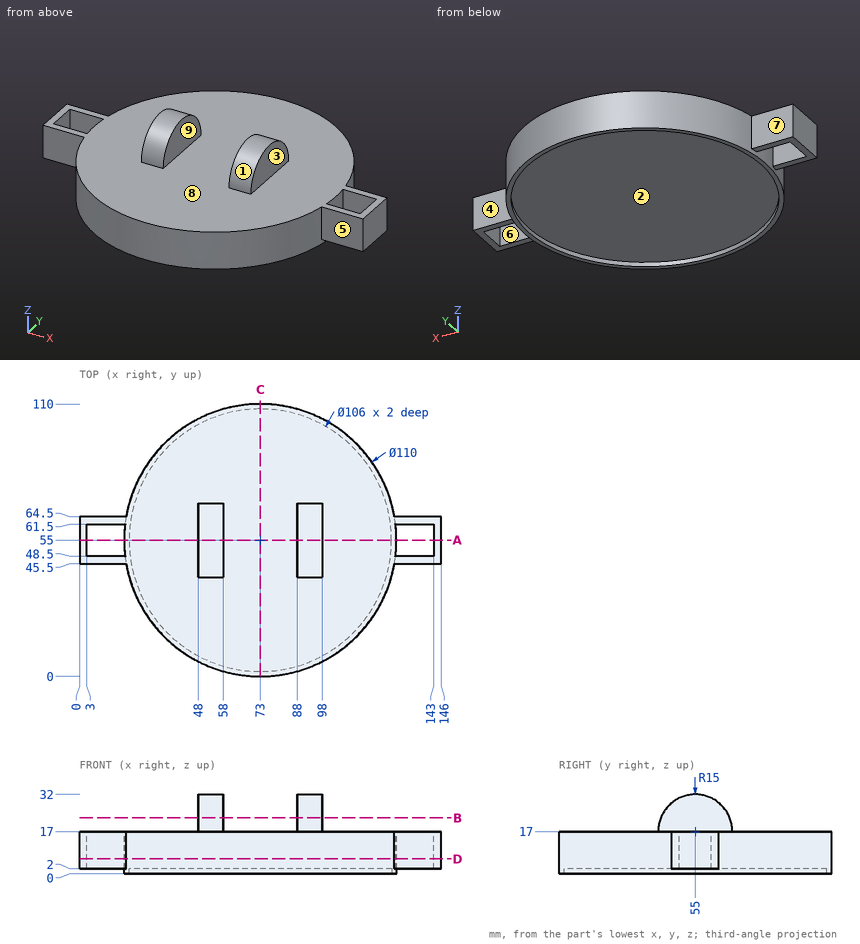
Geometry: see drawing. Coordinates: mm, zero at the bounding-box minimum. A direction names the side the tool comes from. Coordinates: 2 decimals unless noted, no trailing zeros. Write each loop counter-clockwise with the first axis right and the second up, starting at its lowest first coordinate (ties: lowest second). Pieces come first, ordered by that corner, then holes.
1) Section C-C on x = 73. Output: boundary loops of the cut face in (y, z).
2) Section B-B on z = 22.5. Output: boundary loops of the cut face in (x, y).
3) Section D-D on z = 6. Output: boundary loops of the cut face in (x, y), and give its area (3 significant figures).
4) Set-up query: the marked faces 5, 6, 7, 8 and 9. Return all of +Z, -Z, +X, -X, +Y, -Y with unobstructed straight access to the full face (end or side cutting, diameter ignored); none if empty.
5) Material intervals for line 1 along Y through (x, z) = (73, 1); line 2 along X through (y, z) = (42, 19.5); line 3 along Z through (x, y) = (69.5, 97.5), sorted ascending.
6) Pin query (flat end, axial travel): pin 1 Ø4 at (x, y) = (34.5, 28) entering from +Z; pin 2 Ø4.5 at (y, z) = (58.5, 22) entering from +X; pin 3 Ø16.5 at (y, z) = (51.5, 28) entering from -X; pin 4 Ø10.5 at (y, z) = (57.5, 13) entering from -X. Return the tip coordinate at first contact, or that it passes through.
7) Mould query, pull axis Y, two halves, no side actions, for the marked faces 1, 2, 3 and 4. Classes: pulls with the +Y half, pulls with the -Y half, needs draft (parallel to the pull), parting line crosses it, or undercut.
8) Section A-A on y = 55. Output: boundary loops of the cut face in (x, z).
Check result:
1. outline: (0, 0) - (2, 0) - (2, 2) - (108, 2) - (108, 0) - (110, 0) - (110, 17) - (0, 17) - close
2. outline: (48, 41.04) - (58, 41.04) - (58, 68.96) - (48, 68.96) - close; (88, 41.04) - (98, 41.04) - (98, 68.96) - (88, 68.96) - close
3. outline: (0, 45.5) - (18.83, 45.5) arc R55 ccw to (127.17, 45.5) - (146, 45.5) - (146, 64.5) - (127.17, 64.5) arc R55 ccw to (18.83, 64.5) - (0, 64.5) - close; hole (3, 48.5) - (18.39, 48.5) arc R55 cw to (18.39, 61.5) - (3, 61.5) - close; hole (127.61, 48.5) - (143, 48.5) - (143, 61.5) - (127.61, 61.5) arc R55 cw to start
3. area: 9,800 mm2
4. face 5: +Z, -Z, +X, -Y
4. face 6: +Z, -Z
4. face 7: +Z, -Z, -X, +Y
4. face 8: +Z
4. face 9: +Z, +Y, -Y
5. line 1: y = 0 to 2, 108 to 110
5. line 2: x = 48 to 58, 88 to 98
5. line 3: z = 2 to 17
6. pin 1: stops at z = 17
6. pin 2: stops at x = 98
6. pin 3: stops at x = 48
6. pin 4: stops at x = 0
7. face 1: parting line crosses it
7. face 2: undercut
7. face 3: needs draft
7. face 4: pulls with the +Y half
8. outline: (0, 2) - (3, 2) - (3, 17) - (0, 17) - close; (18, 0) - (20, 0) - (20, 2) - (126, 2) - (126, 0) - (128, 0) - (128, 17) - (98, 17) - (98, 32) - (88, 32) - (88, 17) - (58, 17) - (58, 32) - (48, 32) - (48, 17) - (18, 17) - close; (143, 2) - (146, 2) - (146, 17) - (143, 17) - close
